```python
from build123d import *

# Parameters (mm, degrees)
SKETCH1_R           = 29.845
SKETCH1_R_2         = 24.765
BOSS_EXTRUDE1_DEPTH = 97.07
SKETCH4_R           = 24.765
SKETCH4_R_2         = 5.05
CUT_EXTRUDE1_DEPTH  = 95


with BuildPart() as part:
    # Sketch1 → Boss-Extrude1 (new body)
    with BuildSketch(Plane(origin=(0, 0, 0), x_dir=(1, 0, 0), z_dir=(0, 1, 0))):
        with Locations(Location((0, 0, 0), (0, 0, 270))):
            Circle(SKETCH1_R)
        with Locations(Location((0, 0, 0), (0, 0, 270))):
            Circle(SKETCH1_R_2, mode=Mode.SUBTRACT)
    extrude(amount=BOSS_EXTRUDE1_DEPTH)

    # Sketch3 → Revolve1 (revolve)
    with BuildSketch(Plane.XY, mode=Mode.PRIVATE) as revolve1_sk:
        with BuildLine():
            Line((67.945, 0), (29.845, 0))
            Line((29.845, 0), (29.845, 97.07))
            ThreePointArc((29.845, 97.07), (39.711046991, 44.930296079), (67.945, 0))
        make_face()
    revolve(revolve1_sk.sketch.rotate(Axis((0, 0, 0), (0, 1, 0)), 90), axis=Axis((0, 0, 0), (0, 1, 0)))

    # Sketch4 → Cut-Extrude1 (cut)
    with BuildSketch(Plane.XZ):
        with Locations(Location((0, 0, 0), (0, 0, 90))):
            Circle(SKETCH4_R)
        with Locations(Location((0, 55.245, 0), (0, 0, 270))):
            Circle(SKETCH4_R_2)
        with Locations(Location((47.843573432, -27.6225, 0), (0, 0, 270))):
            Circle(SKETCH4_R_2)
        with Locations(Location((-47.843573432, -27.6225, 0), (0, 0, 270))):
            Circle(SKETCH4_R_2)
    extrude(amount=-CUT_EXTRUDE1_DEPTH, mode=Mode.SUBTRACT)


solid = part.part
```
Check sheet for the modelled part. Datum: model origin and axes. Units: mm. Coordinates: 2 decimals unless noted, no trailing zeros. Write each loop counter-clockwise with the first axis right and the second up, starting at its lowest first coordinate (ties: lowest second). Pieces come first, ordered by that corner, then holes. Notation, with made-up numbers: (64.5, 15.5) -> (104.5, 15.5) arc R23 ccw to (104.5, 45.5) -> close; hole circle Ø2 at (77, 38.25). An arc over 180 degrees is marked (long way). Use a Markdown table: item, result.
1. Release check for a two-part mould opening along X. For faces 1 (the flat face through (18, 97.07, -18)), 2 (the cylindrical face through (-44.43, 9.02, -23.9)) record: pulls with the +X half, pulls with the -X half, needs draft (parallel to the pull), parting line crosses it, or undercut.
Reported:
| item | result |
|---|---|
| face 1 | needs draft |
| face 2 | undercut |
2. Scan lines: line 1 along X through (y, z) = (43.5, -2.5); line 2 along X through (y, z) = (71, 0) (3 decimals); line 3 along Z through (x, y) = (17, 60). Record each from-to range of solid material in increasing order.
Reported:
| item | result |
|---|---|
| line 1 | x = -40.2 to -24.64, 24.64 to 40.2 |
| line 2 | x = -32.246 to -24.765, 24.765 to 32.246 |
| line 3 | z = -30.3 to -18.01, 18.01 to 30.3 |
3. Go/stop test with flat-tipped pins: pin 1 Ø3 at (y, z) = (44, 13) entering from +X; pin 2 Ø1 at (y, z) = (69.5, 28) entering from -X; pin 3 Ø1 at (x, z) = (-48, -1) entering from +Y. Record where each tip stops, or that it passes through.
Reported:
| item | result |
|---|---|
| pin 1 | stops at x = 38.72 |
| pin 2 | stops at x = -17.4 |
| pin 3 | stops at y = 28.3 |
4. Sectioned sample at D-D (y = 38.5). Enter the section's corners in (x, z) (3 decimals).
Reported:
| item | result |
|---|---|
| outline | circle Ø84.836 at (0, 0); hole circle Ø49.53 at (0, 0) |
5. Sectioned sample at A-A (z = 0). Enter the section's corners in (x, y) (3 decimals).
Reported:
| item | result |
|---|---|
| outline | (-67.945, 0) -> (-24.765, 0) -> (-24.765, 97.07) -> (-29.845, 97.07) arc R142.706 cw to start; (24.765, 0) -> (67.945, 0) arc R142.706 cw to (29.845, 97.07) -> (24.765, 97.07) -> close |
6. Sectioned sample at C-C (z = -28). Give the number of separate pieces and of enclosed holes in the cut face, plus the area to 3 significant figures.
Reported:
| item | result |
|---|---|
| separate pieces | 3 |
| enclosed holes | 0 |
| area | 5,350 mm2 |
